Print and shaded views of the part. All mm, measured from the part's lowest x, y and z. Round coordinates to 2 decimals unless told otherwise and drop trailing zeros. Write each loop counter-clockwise with the first axis right and the second up, starting at its lowest first coordinate (ties: lowest second). Pieces come first, ordered by that corner, then holes. Notation, with made-up numbers: M 70.25,44.5 L 100.25,44.5 A31 ccw 100.25,68.5 Z; hole C -34.75,-34.5 d11. An arc over 180 degrees is marked long. Write item = value, one per line. Start each with the question number.
Q1. Drop flat-ended pins along their axis: P1, Ø1.2, axis at y = 2.5, z = 43, coming from the -X side; P2, Ø1.2, axis at y = 1.5, z = 40.5, coming from the +X side; P3, Ø1.1, axis at x = 3, z = 3, coming from the +Y side; P4, Ø2, axis at x = 16.5, y = 2, coming from the +Z side. Give the stop position or say it passes through.
Q2. Band-saw the part on D-D on z = 63. Write the cut outline in (x, y), plus the area to 3 significant figures.
Q3. Band-saw the part on C-C on x = 32.5. Write the cut outline in (y, z).
Q4. Band-saw the part on B-B on z = 39.5. Write the cut outline in (x, y).
Q5. Probe L1, parallel to Z at x = 15.5, y = 2.65; L2, parallel to X at y = 2.3, z = 11.5; L3, parallel to X at y = 3.55, z = 63. List the from-to ranges inside material, lowest first.
Q6. Band-saw the part on A-A on x = 21.5. Write the cut outline in (y, z).
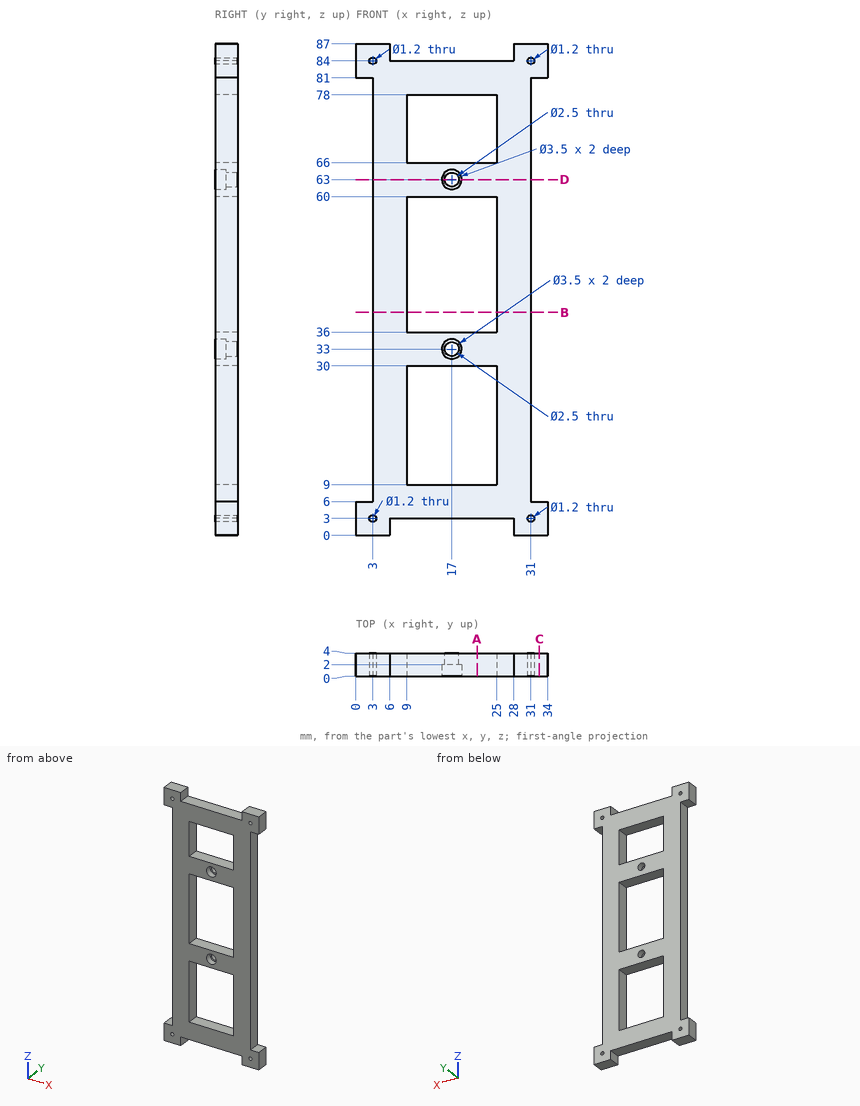
Conclusion:
q1.P1 = 3
q1.P2 = 31
q1.P3 = through
q1.P4 = 84
q2.outline = M 3,0 L 15.25,0 L 15.25,2 L 15.75,2 L 15.75,4 L 3,4 Z; M 18.25,2 L 18.75,2 L 18.75,0 L 31,0 L 31,4 L 18.25,4 Z
q2.area = 100 mm^2
q3.outline = M 0,0 L 4,0 L 4,6 L 0,6 Z; M 0,81 L 4,81 L 4,87 L 0,87 Z
q4.outline = M 3,0 L 9,0 L 9,4 L 3,4 Z; M 25,0 L 31,0 L 31,4 L 25,4 Z
q5.L1 = 3 to 9, 30 to 36, 60 to 66, 78 to 84
q5.L2 = 3 to 9, 25 to 31
q5.L3 = 3 to 15.75, 18.25 to 31
q6.outline = M 0,3 L 4,3 L 4,9 L 0,9 Z; M 0,30 L 4,30 L 4,36 L 0,36 Z; M 0,60 L 4,60 L 4,66 L 0,66 Z; M 0,78 L 4,78 L 4,84 L 0,84 Z
